Autodesk Inventor part; units mm, degrees
ref_plane "YZ Plane" through (0, 0, 0) normal (1, 0, 0) x (0, 1, 0)
ref_plane "XZ Plane" through (0, 0, 0) normal (0, 1, 0) x (-1, 0, 0)
ref_plane "XY Plane" through (0, 0, 0) normal (0, 0, 1) x (1, 0, 0)
sketch "スケッチ1" plane through (0, 0, 0) normal (0, 0, 1) x (1, 0, 0)
  line L0 (-57.6728, -0.0614) -> (72.3272, -0.0614)
  line L1 (72.3272, -0.0614) -> (72.3272, -22.0614)
  line L2 (72.3272, -22.0614) -> (-57.6728, -22.0614)
  line L3 (-57.6728, -22.0614) -> (-57.6728, -0.0614)
  circle A0 centre (-25.1728, -11.0614) radius 6
  circle A1 centre (39.8272, -11.0614) radius 6
  line L4 (-21.2046, -6.5611) -> (35.8589, -6.5611)
  line L5 (-21.2046, -15.5617) -> (35.8589, -15.5617)
  point P0 (0, 0)
  dimension "d0" = 130
  dimension "d1" = 22
  dimension "d4" = 12
  dimension "d5" = 12
  dimension "d6" = 65
  dimension "d7" = 11
  dimension "d8" = 11
  dimension "d9" = 32.5
extrude "押し出し1" add sketch "スケッチ1" along normal blind 30 contours L0 L1 L2 L3 | A0 | A0 L4 A1 L5 | A1
extrude "押し出し2" cut sketch "スケッチ1" along normal blind 30 contours A0 | A0 L4 A1 L5 | A1
sketch "スケッチ2" plane through (-57.6728, -0.0614, 0) normal (0, 1, 0) x (1, 0, 0)
  circle A0 centre (12, -7.5) radius 3
  line L0 (65, -1.1982) -> (65, -25.359)
  line L1 (8.4096, -15) -> (24.5168, -15)
  line L2 (130, 0) -> (130, -30)
  line L3 (0, 0) -> (130, 0)
  line L4 (0, 0) -> (0, -30)
  circle A1 centre (12, -22.5) radius 3
  circle A2 centre (118, -7.5) radius 3
  circle A3 centre (118, -22.5) radius 3
  point P0 (57.6728, 0)
  dimension "d12" = 6
  dimension "d13" = 65
  dimension "d14" = 15
  dimension "d15" = 12
  dimension "d16" = 7.5
hole "穴1" at (-45.6728, -0.0614, 7.5) at (-45.6728, -0.0614, 22.5) at (60.3272, -0.0614, 7.5) at (60.3272, -0.0614, 22.5) direction (0, -1, 0) diameter 4.917 end through all
properties part number "sc601_load_cell" material "アルミニウム 6061-O"
Here's how the part is built. I have some questions about the finished solid (model axes, mm). A direction names the side the tool comes from. Coordinates: 2 decimals unless noted, no trailing zeros. Loops run counter-clockwise (first coordinate to the right, second up) from the corner with the lowest first, then second, coordinate; pieces in that order, holes last. Notation, with made-up numbers: (-33.75, 61.25) -> (-17.75, 61.25) arc R27 ccw to (-17.75, 80.25) -> close; hole circle Ø4 at (-15.5, 21.5). An arc over 180 degrees is marked (long way). Use one line per item in the form item = value. Start each with the question number.
(1) If we section it at C-C (x = 44.5): Please give me the cut outline in (y, z).
(2) On a 3-axis mill with a long thin cutter (end or side, diameter ignored), from which of +Z, -Z, +X, -X, +Y, -Y can I reach the whole of each face in a straight line? I mean faces 1 (the face through (7, -6.561, 15)), 2 (the face through (72.327, -11, 15)). Say none if no direction works.
(3) Please list where these lines run through material, in increasing order: line 1 along X through (y, z) = (-10.5, 22.5); line 2 along X through (y, z) = (-5, 7.5); line 3 along Y through (x, z) = (-25.5, 15.25).
(4) Will this pin go through, and if not, where does the flat tip stop? pin 1 (4.5 mm diameter, centred on x = 60.33, z = 7.5, fed in from +Y).
(5) If we section it at B-B (x = -17): Please give me the cut outline in (y, z), then the cut area to 3 significant figures.
(6) We'd pull the mould along Z, two halves only. Please class faces 3 (the face through (6, -16, 30)), 4 (the face through (8, -22.061, 15)), 5 (the face through (-43.49, -11.22, 8.63)): pulls with the +Z half, pulls with the -Z half, needs draft (parallel to the pull), parting line crosses it, or undercut.
(7) If we section it at A-A (z = 7.5): Please give me the cut outline in (x, y), then the cut area to 3 significant figures.
Verdict:
q1.outline = (-22.06, 0) -> (-14.83, 0) -> (-14.83, 30) -> (-22.06, 30) -> close; (-7.3, 0) -> (-0.06, 0) -> (-0.06, 30) -> (-7.3, 30) -> close
q2.face_1 = +Z, -Z
q2.face_2 = +Z, -Z, +X, +Y, -Y
q3.line_1 = -57.67 to -48.13, -43.21 to -31.15, 45.8 to 57.87, 62.79 to 72.33
q3.line_2 = -57.67 to -48.13, -43.21 to 57.87, 62.79 to 72.33
q3.line_3 = -22.06 to -17.05, -5.07 to -0.06
q4.pin_1 = through
q5.outline = (-22.06, 0) -> (-15.56, 0) -> (-15.56, 30) -> (-22.06, 30) -> close; (-6.56, 0) -> (-0.06, 0) -> (-0.06, 30) -> (-6.56, 30) -> close
q5.area = 390 mm²
q6.face_3 = pulls with the +Z half
q6.face_4 = needs draft
q6.face_5 = undercut
q7.outline = (-57.67, -22.06) -> (-48.13, -22.06) -> (-48.13, -0.06) -> (-57.67, -0.06) -> close; (-43.21, -22.06) -> (57.87, -22.06) -> (57.87, -0.06) -> (-43.21, -0.06) -> close; (62.79, -22.06) -> (72.33, -22.06) -> (72.33, -0.06) -> (62.79, -0.06) -> close; hole (-21.2, -15.56) -> (35.86, -15.56) arc R6 ccw (long way) to (35.86, -6.56) -> (-21.2, -6.56) arc R6 ccw (long way) to start
q7.area = 1,930 mm²
